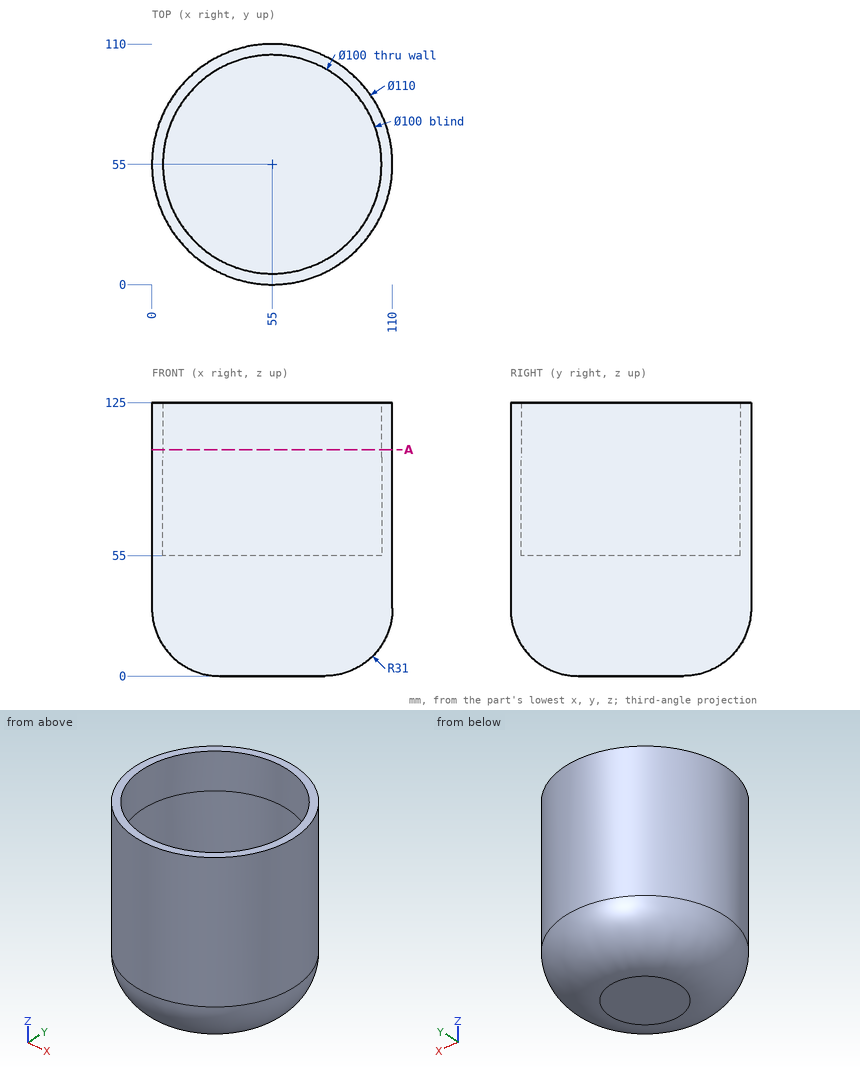
Verification items for this drawing (mm, ordinates from the low corner). Coordinates: 2 decimals unless noted, no trailing zeros. Order: outer loops, then holes, each group sorted by start corner. A loop starts at its lowest first (then second) coordinate and runs counter-clockwise, first axis right, second up. Notation, with made-up numbers: (-35.75, 35.5) - (-3.75, 35.5) arc R28 ccw to (-3.75, 71.5) - close; hole circle Ø3 at (69, 13). An arc over 180 degrees is marked (long way). Use one line per item in the form item = value.
1. Section check A-A (z = 103.5). Record the boundary of the cut face in (x, y), then the cut area to 3 significant figures.
Here are the results:
outline = circle Ø110 at (55, 55); hole circle Ø100 at (55, 55)
area = 1,650 mm²
2. Gauge pin test, flat ends, axial feed: pin 1 (8 mm diameter, centred on x = 17.5, y = 95.5, fed in from -Z); pin 2 (12 mm diameter, centred on x = 87, z = 66.5, fed in from -Y); pin 3 (12 mm diameter, centred on x = 17.5, z = 41.5, fed in from -Y). Record the tip position at first contact, or that the pin passes through.
Here are the results:
pin_1 = 16.12
pin_2 = 6.53
pin_3 = 9.91
3. Scan lines: line 1 (Y direction, x = 55, z = 113.25); line 2 (X direction, y = 88, z = 97.5); line 3 (Z direction, x = 33, y = 52.5). Record each from-to range of solid material in increasing order.
Here are the results:
line_1 = 0 to 5, 105 to 110
line_2 = 11 to 17.44, 92.56 to 99
line_3 = 0 to 55
